```python
from build123d import *

# Parameters (mm, degrees)
F0_W           = 12
F0_H           = 25
F0_R           = 2.5
F1_DEPTH       = 5
F3_D           = 3
F3_CSINK_D     = 7.5
F3_CSINK_ANGLE = 90


with BuildPart() as f1:
    # F0 (on Top) → F1 (new body)
    with BuildSketch(Plane.XY):
        Rectangle(F0_W, F0_H)
        Circle(F0_R, mode=Mode.SUBTRACT)
    extrude(amount=F1_DEPTH)

    # F3 (through all)
    with Locations(Plane(origin=(0, 0, 0), x_dir=(1, 0, 0), z_dir=(0, 0, -1))):
        with Locations((0, 7.5), (0, -7.5)):
            CounterSinkHole(F3_D / 2, F3_CSINK_D / 2, counter_sink_angle=F3_CSINK_ANGLE)


solid = f1.part
```
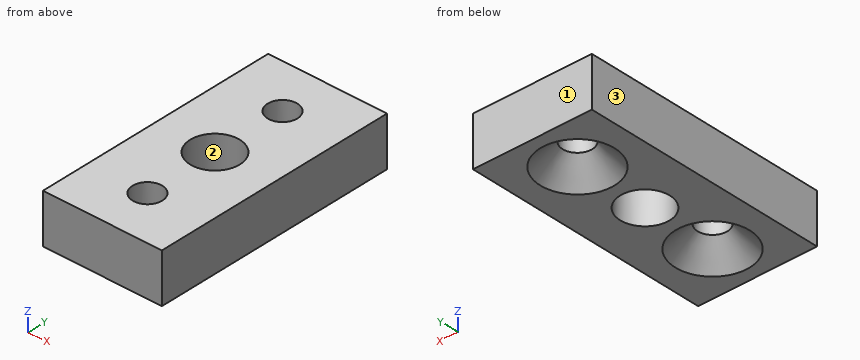
Here's how the part is built. I have some questions about the finished solid (model axes, mm). Face numbers are marked on the shaded views. Coordinates: 2 decimals unless noted, no trailing zeros. Order: outer loops, then holes, each group sorted by start corner. A loop starts at its lowest first (then second) coordinate and runs counter-clockwise, first axis right, second up. Notation, with made-up numbers: M 32.5,88 L 88.5,88 A24 cw 88.5,123 Z; hole C 26.5,10 d1. An arc over 180 degrees is marked long. Answer as a JSON object with one key per item and string values. Group by question number.
(1) I need wall thicknesses on probe 1 along Y at (x, z) = (0, 3.8); probe 2 along X at (y, z) = (7.5, 4.1); probe 3 along Y at (x, z) = (1, 0.4). Which ranges of each line are inside material? Lowest first, please.
(2) Suppose I cut it at D-D, the plane z = 1.45. Please give me the cut outline in (x, y), then the cut area to 3 significant figures.
(3) Suppose I cut it at C-C, the plane y = -7.5. Please give me the cut outline in (x, z).
(4) If we mould it in two halves opening along Y, with no side actions, what happens to the marked faces 1, 2 and 3? For each: released by +Y, released by -Y, zero draft, split by the parting line, or undercut.
(5) Suppose I cut it at A-A, the plane x = 0. Please give me the cut outline in (y, z), then the cut area to 3 significant figures.
(6) Suppose I cut it at B-B, the plane z = 3.9. Please give me the cut outline in (x, y), then the cut area to 3 significant figures.
Values found:
{
 "1": {"probe 1": "y = -12.5 to -9, -6 to -2.5, 2.5 to 6, 9 to 12.5", "probe 2": "x = -6 to -1.5, 1.5 to 6", "probe 3": "y = -12.5 to -10.7, -4.3 to -2.29, 2.29 to 4.3, 10.7 to 12.5"},
 "2": {"outline": "M -6,-12.5 L 6,-12.5 L 6,12.5 L -6,12.5 Z; hole C 0,0 d5; hole C 0,-7.5 d4.6; hole C 0,7.5 d4.6", "area": "247 mm^2"},
 "3": {"outline": "M -6,0 L -3.75,0 L -1.5,2.25 L -1.5,5 L -6,5 Z; M 1.5,2.25 L 3.75,0 L 6,0 L 6,5 L 1.5,5 Z"},
 "4": {"face 1": "released by +Y", "face 2": "undercut", "face 3": "zero draft"},
 "5": {"outline": "M -12.5,0 L -11.25,0 L -9,2.25 L -9,5 L -12.5,5 Z; M -6,2.25 L -3.75,0 L -2.5,0 L -2.5,5 L -6,5 Z; M 2.5,0 L 3.75,0 L 6,2.25 L 6,5 L 2.5,5 Z; M 9,2.25 L 11.25,0 L 12.5,0 L 12.5,5 L 9,5 Z", "area": "59.9 mm^2"},
 "6": {"outline": "M -6,-12.5 L 6,-12.5 L 6,12.5 L -6,12.5 Z; hole C 0,0 d5; hole C 0,-7.5 d3; hole C 0,7.5 d3", "area": "266 mm^2"}
}
